Here's how the part is built. I have some questions about the finished solid (model axes, mm). Face numbers are marked on the shaded views. Round coordinates to 2 decimals unless told otherwise and drop trailing zeros. Loops run counter-clockwise (first coordinate to the right, second up) from the corner with the lowest first, then second, coordinate; pieces in that order, holes last. Notation, with made-up numbers: M 61,73.25 L 77,73.25 A22 ccw 77,88.25 Z; hole C 17,78 d5. An arc over 180 degrees is marked long. Use a Markdown table: item, result.
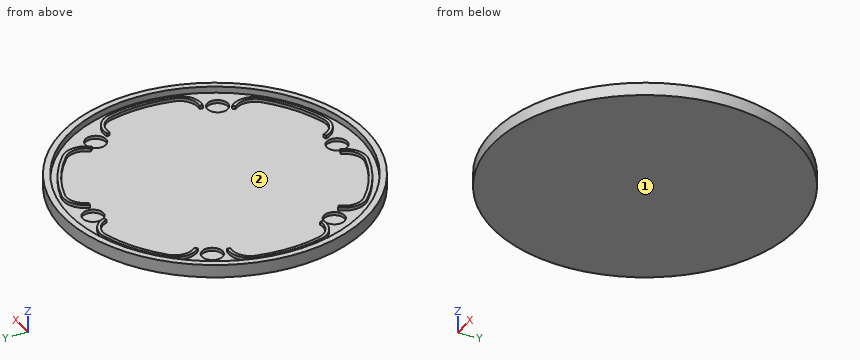
Autodesk Inventor part; units mm, degrees
ref_plane "YZ Plane" through (0, 0, 0) normal (1, 0, 0) x (0, 1, 0)
ref_plane "XZ Plane" through (0, 0, 0) normal (0, 1, 0) x (-1, 0, 0)
ref_plane "XY Plane" through (0, 0, 0) normal (0, 0, 1) x (1, 0, 0)
sketch "Sketch3" plane through (0, 0, 0) normal (0, 0, 1) x (1, 0, 0)
  circle A0 centre (0, 0) radius 68
  circle A1 centre (0, 0) radius 65
  circle A2 centre (0, 0) radius 71
  dimension "d27" = 136
  dimension "d28" = 130
  dimension "d29" = 142
extrude "Extrusion3" add sketch "Sketch3" along normal blind 3 contours A0 | A1 | A2
sketch "Sketch4" plane through (0, 0, 3) normal (0, 0, 1) x (1, 0, 0)
  circle A0 centre (0, 0) radius 71
  line L0 (0, 0) -> (0, 63.1147) construction
  circle A1 centre (0, 57.5) radius 4.8
  circle A2 centre (-49.7965, 28.75) radius 4.8
  circle A3 centre (-49.7965, -28.75) radius 4.8
  circle A4 centre (0, -57.5) radius 4.8
  circle A5 centre (49.7965, -28.75) radius 4.8
  circle A6 centre (49.7965, 28.75) radius 4.8
  dimension "d32" = 9.6
  dimension "d33" = 57.5
  dimension "d36" = 360
extrude "Extrusion4" cut sketch "Sketch4" against normal blind 1.524 contours A1 | A2 | A3 | A4 | A5 | A6
sketch "Sketch5" plane through (0, 0, 3) normal (0, 0, 1) x (1, 0, 0)
  circle A0 centre (49.7965, -28.75) radius 4.8
  circle A1 centre (-49.7965, 28.75) radius 4.8
  circle A2 centre (49.7965, 28.75) radius 4.8
  circle A3 centre (0, -57.5) radius 4.8
  circle A4 centre (-49.7965, -28.75) radius 4.8
  circle A5 centre (0, 57.5) radius 4.8
  circle A6 centre (0, 0) radius 71
  circle A7 centre (0, 57.5) radius 6.3
  circle A8 centre (-49.7965, 28.75) radius 6.3
  circle A9 centre (-49.7965, -28.75) radius 6.3
  circle A10 centre (0, -57.5) radius 6.3
  circle A11 centre (49.7965, -28.75) radius 6.3
  circle A12 centre (49.7965, 28.75) radius 6.3
  circle A13 centre (0, 0) radius 65
  circle A14 centre (-15.5907, 52.744) radius 10
  circle A15 centre (15.5907, 52.744) radius 10
  circle A16 centre (-37.8823, 39.874) radius 10
  circle A17 centre (-53.473, 12.87) radius 10
  circle A18 centre (-53.473, -12.87) radius 10
  circle A19 centre (-37.8823, -39.874) radius 10
  circle A20 centre (-15.5907, -52.744) radius 10
  circle A21 centre (15.5907, -52.744) radius 10
  circle A22 centre (37.8823, -39.874) radius 10
  circle A23 centre (53.473, -12.87) radius 10
  circle A24 centre (53.473, 12.87) radius 10
  circle A25 centre (37.8823, 39.874) radius 10
  circle A26 centre (-15.5907, 52.744) radius 8.5
  circle A27 centre (-37.8823, 39.874) radius 8.5
  arc A28 (-18.0002, 60.8953) -> (-43.7368, 46.0363) centre (0, 0) ccw
  line L0 (-45.1916, 33.0494) -> (-44.0952, 34.0731)
  line L1 (-6.0259, 55.6618) -> (-7.4606, 55.2241)
  line L2 (-51.2175, 22.6123) -> (-51.5558, 21.151)
  arc A29 (-61.737, 14.859) -> (-61.737, -14.859) centre (0, 0) ccw
  line L3 (-51.2175, -22.6123) -> (-51.5558, -21.151)
  circle A30 centre (-53.473, -12.87) radius 8.5
  circle A31 centre (-53.473, 12.87) radius 8.5
  line L4 (-45.1916, -33.0494) -> (-44.0952, -34.0731)
  arc A32 (-43.7368, -46.0363) -> (-18.0002, -60.8953) centre (0, 0) ccw
  line L5 (-6.0259, -55.6618) -> (-7.4606, -55.2241)
  circle A33 centre (-15.5907, -52.744) radius 8.5
  circle A34 centre (-37.8823, -39.874) radius 8.5
  line L6 (6.0259, -55.6618) -> (7.4606, -55.2241)
  arc A35 (18.0002, -60.8953) -> (43.7368, -46.0363) centre (0, 0) ccw
  line L7 (45.1916, -33.0494) -> (44.0952, -34.0731)
  circle A36 centre (37.8823, -39.874) radius 8.5
  circle A37 centre (15.5907, -52.744) radius 8.5
  line L8 (51.2175, -22.6123) -> (51.5558, -21.151)
  arc A38 (61.737, -14.859) -> (61.737, 14.859) centre (0, 0) ccw
  line L9 (51.2175, 22.6123) -> (51.5558, 21.151)
  circle A39 centre (53.473, 12.87) radius 8.5
  circle A40 centre (53.473, -12.87) radius 8.5
  line L10 (45.1916, 33.0494) -> (44.0952, 34.0731)
  arc A41 (43.7368, 46.0363) -> (18.0002, 60.8953) centre (0, 0) ccw
  line L11 (6.0259, 55.6618) -> (7.4606, 55.2241)
  circle A42 centre (15.5907, 52.744) radius 8.5
  circle A43 centre (37.8823, 39.874) radius 8.5
  point P0 (-63.1954, 15.2101)
  point P1 (-63.1954, -15.2101)
  point P2 (-45.1916, -33.0494)
  point P3 (-44.77, -47.1238)
  point P4 (-18.4254, -62.3338)
  point P5 (-6.0259, -55.6618)
  point P6 (6.0259, -55.6618)
  point P7 (18.4254, -62.3338)
  point P8 (44.77, -47.1238)
  point P9 (45.1916, -33.0494)
  point P10 (63.1954, -15.2101)
  point P11 (63.1954, 15.2101)
  point P12 (51.2175, 22.6123)
  point P13 (45.1916, 33.0494)
  point P14 (44.77, 47.1238)
  point P15 (18.4254, 62.3338)
  point P16 (6.0259, 55.6618)
  point P17 (-18.4254, 62.3338)
  point P18 (-44.77, 47.1238)
  dimension "d46" = 20
  dimension "d40" = 1.5
  dimension "d43" = 360
  dimension "d45" = 130
  dimension "d47" = 20
  dimension "d50" = 360
  dimension "d52" = 1.5
  dimension "d53" = 1.5
  dimension "d56" = 360
extrude "Extrusion5" add sketch "Sketch5" along normal blind 1.5 contours L1 A26 A28 A14 | A15 A41 A42 L11 | A14 A28 A16 A13 | A13 A25 A41 A15 | A16 A28 A27 L0 | A25 L10 A43 A41 | A17 A29 A18 A13 | A17 L2 A31 A29 | A13 A23 A38 A24 | A24 A38 A39 L9 | A18 A29 A30 L3 | A19 A32 A20 A13 | A19 L4 A34 A32 | A23 L8 A40 A38 | A20 A32 A33 L5 | A13 A21 A35 A22 | A22 A35 A36 L7 | A21 L6 A37 A35 picked at (-10.8394, 60.9083) picked at (10.8394, 60.9083) picked at (-44.9035, 46.1933) picked at (47.256, 41.1158) picked at (-62.4563, 15.7909) picked at (62.2412, 16.3841) picked at (-62.2412, -16.3841) picked at (-45.2691, -33.9863) picked at (62.4563, -15.7909) picked at (-10.8394, -60.9083) picked at (44.8652, -46.2495) picked at (10.8394, -60.9083)
sketch "Sketch6" plane through (0, 0, 3) normal (0, 0, 1) x (1, 0, 0)
  circle A0 centre (0, 0) radius 71
  circle A1 centre (0, 0) radius 68
  dimension "d60" = 136
extrude "Extrusion6" add sketch "Sketch6" along normal blind 3
equation "\"d47\" = d46"
equation "\"d53\" = d52"
properties part number "Bottom Lid"
1. We'd pull the mould along Y, two halves only. Please class the marked faces 1 and 2: +Y half, -Y half, draft (parallel to the pull), parting line (faces both ways), or undercut.
Answer sheet:
| item | result |
|---|---|
| face 1 | draft |
| face 2 | undercut |
2. I need wall thicknesses on probe 1 along Y at (x, z) = (0, 2.45); probe 2 along Y at (x, z) = (-33, 4.3); probe 3 along X at (y, z) = (-56, 3.75). Which ranges of each line are inside material? Lowest first, please. Write a range as from..to.
Answer sheet:
| item | result |
|---|---|
| probe 1 | -71..-62.3, -52.7..52.7, 62.3..71 |
| probe 2 | -62.86..-59.46, -56..-54.25, 54.25..56, 59.46..62.86 |
| probe 3 | -43.65..-38.57, -33..-29.94, -7.74..-6.14, 6.14..7.74, 29.94..33, 38.57..43.65 |
3. Imagine slicing it at B-B, the plane y = 0. Write out the boundary of the cut face in (x, z), then the cut area to 4 significant figures.
Answer sheet:
| item | result |
|---|---|
| outline | M -71,0 L 71,0 L 71,6 L 68,6 L 68,3 L 65,3 L 65,4.5 L 63.5,4.5 L 63.5,3 L -63.5,3 L -63.5,4.5 L -65,4.5 L -65,3 L -68,3 L -68,6 L -71,6 Z |
| area | 448.5 mm2 |
4. For pin 1 Ø11 at (x, y) = (0, -57.5) entering from +Z; pin 2 Ø3 at (y, z) = (-21.5, 5) entering from -X; pin 3 Ø7.5 at (x, y) = (49.8, -28.75) entering from -Z; pin 4 Ø1 at (y, z) = (40.5, 4) entering from +X, each with a flat end and sliding along its axis, tell me the tip position at first contact or that it passes through.
Answer sheet:
| item | result |
|---|---|
| pin 1 | z = 3 |
| pin 2 | x = -68.12 |
| pin 3 | z = 0 |
| pin 4 | x = 58.66 |
5. Imagine slicing it at C-C, the plane y = 57.5. Write out the boundary of the cut face in (x, z), then the cut area to 3 significant figures.
Answer sheet:
| item | result |
|---|---|
| outline | M -41.65,0 L 41.65,0 L 41.65,6 L 36.3,6 L 36.3,3 L 30.31,3 L 30.31,4.5 L 26.94,4.5 L 26.94,3 L 8.55,3 L 8.55,4.5 L 6.79,4.5 L 6.79,3 L 4.8,3 L 4.8,1.48 L -4.8,1.48 L -4.8,3 L -6.79,3 L -6.79,4.5 L -8.55,4.5 L -8.55,3 L -26.94,3 L -26.94,4.5 L -30.31,4.5 L -30.31,3 L -36.3,3 L -36.3,6 L -41.65,6 Z |
| area | 283 mm2 |
6. Imagine slicing it at A-A, the plane x = 0. Write out the boundary of the cut face in (y, z).
Answer sheet:
| item | result |
|---|---|
| outline | M -71,0 L 71,0 L 71,6 L 68,6 L 68,3 L 62.3,3 L 62.3,1.48 L 52.7,1.48 L 52.7,3 L -52.7,3 L -52.7,1.48 L -62.3,1.48 L -62.3,3 L -68,3 L -68,6 L -71,6 Z |
